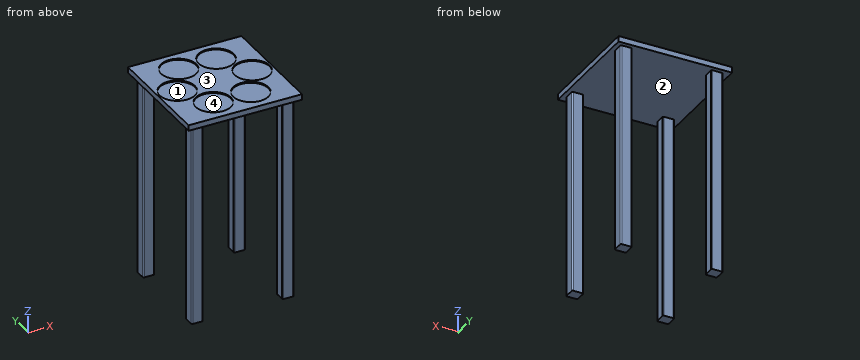
from build123d import *

# Parameters (mm, degrees)
F0_W     = 500
F0_H     = 500
F0_R     = 77.5
F1_DEPTH = 25
F2_DEPTH = 5
F4_DEPTH = 900


with BuildPart() as f1:
    # F0 (on Top) → F1 (new body)
    with BuildSketch(Plane.XY):
        with Locations((0, -2.197117)):
            Rectangle(F0_W, F0_H)
        with Locations((-82.5, -142.894192)):
            Circle(F0_R, mode=Mode.SUBTRACT)
        with Locations((82.5, -142.894192)):
            Circle(F0_R, mode=Mode.SUBTRACT)
        with Locations((-165, 0)):
            Circle(F0_R, mode=Mode.SUBTRACT)
        with Locations((-82.5, 142.894192)):
            Circle(F0_R, mode=Mode.SUBTRACT)
        with Locations((165, 0)):
            Circle(F0_R, mode=Mode.SUBTRACT)
        with Locations((82.5, 142.894192)):
            Circle(F0_R, mode=Mode.SUBTRACT)
        with Locations((-82.5, 142.894192)):
            Circle(F0_R)
        with Locations((82.5, 142.894192)):
            Circle(F0_R)
        with Locations((165, 0)):
            Circle(F0_R)
        with Locations((-165, 0)):
            Circle(F0_R)
        with Locations((-82.5, -142.894192)):
            Circle(F0_R)
        with Locations((82.5, -142.894192)):
            Circle(F0_R)
    extrude(amount=-F1_DEPTH)

    # F0 (on Top) → F2 (cut)
    with BuildSketch(Plane.XY):
        with Locations((-82.5, 142.894192)):
            Circle(F0_R)
        with Locations((82.5, 142.894192)):
            Circle(F0_R)
        with Locations((165, 0)):
            Circle(F0_R)
        with Locations((82.5, -142.894192)):
            Circle(F0_R)
        with Locations((-82.5, -142.894192)):
            Circle(F0_R)
        with Locations((-165, 0)):
            Circle(F0_R)
    extrude(amount=-F2_DEPTH, mode=Mode.SUBTRACT)

    # F3 (on face) → F4 (join)
    with BuildSketch(Plane(origin=(0, 0, -25), x_dir=(1, 0, 0), z_dir=(0, 0, -1))):
        with BuildLine():
            ThreePointArc((225, 172.197117), (228.535534, 173.661583), (230, 177.197117))
            Line((230, 177.197117), (230, 217.197117))
            ThreePointArc((230, 217.197117), (228.535534, 220.732651), (225, 222.197117))
            Line((225, 222.197117), (185, 222.197117))
            ThreePointArc((185, 222.197117), (181.464466, 220.732651), (180, 217.197117))
            Line((180, 217.197117), (180, 177.197117))
            ThreePointArc((180, 177.197117), (181.464466, 173.661583), (185, 172.197117))
            Line((185, 172.197117), (225, 172.197117))
        make_face()
        with BuildLine():
            ThreePointArc((-175, 172.197117), (-171.464466, 173.661583), (-170, 177.197117))
            Line((-170, 177.197117), (-170, 217.197117))
            ThreePointArc((-170, 217.197117), (-171.464466, 220.732651), (-175, 222.197117))
            Line((-175, 222.197117), (-215, 222.197117))
            ThreePointArc((-215, 222.197117), (-218.535534, 220.732651), (-220, 217.197117))
            Line((-220, 217.197117), (-220, 177.197117))
            ThreePointArc((-220, 177.197117), (-218.535534, 173.661583), (-215, 172.197117))
            Line((-215, 172.197117), (-175, 172.197117))
        make_face()
        with BuildLine():
            ThreePointArc((-175, -227.802883), (-171.464466, -226.338417), (-170, -222.802883))
            Line((-170, -222.802883), (-170, -182.802883))
            ThreePointArc((-170, -182.802883), (-171.464466, -179.267349), (-175, -177.802883))
            Line((-175, -177.802883), (-215, -177.802883))
            ThreePointArc((-215, -177.802883), (-218.535534, -179.267349), (-220, -182.802883))
            Line((-220, -182.802883), (-220, -222.802883))
            ThreePointArc((-220, -222.802883), (-218.535534, -226.338417), (-215, -227.802883))
            Line((-215, -227.802883), (-175, -227.802883))
        make_face()
        with BuildLine():
            Line((185, -227.802883), (225, -227.802883))
            ThreePointArc((225, -227.802883), (228.535534, -226.338417), (230, -222.802883))
            Line((230, -222.802883), (230, -182.802883))
            ThreePointArc((230, -182.802883), (228.535534, -179.267349), (225, -177.802883))
            Line((225, -177.802883), (185, -177.802883))
            ThreePointArc((185, -177.802883), (181.464466, -179.267349), (180, -182.802883))
            Line((180, -182.802883), (180, -222.802883))
            ThreePointArc((180, -222.802883), (181.464466, -226.338417), (185, -227.802883))
        make_face()
    extrude(amount=F4_DEPTH)


solid = f1.part
CAD build for the part. Positions are in the model's coordinates, mm. Face numbers are marked on the shaded views. A direction names the side the tool comes from. Round coordinates to 2 decimals unless told otherwise and drop trailing zeros. Order: outer loops, then holes, each group sorted by start corner. A loop starts at its lowest first (then second) coordinate and runs counter-clockwise, first axis right, second up. Notation, with made-up numbers: (-4, 44) -> (17, 44) arc R22 cw to (17, 60) -> close; hole circle Ø2 at (-39.75, 0.5). An arc over 180 degrees is marked (long way). Write each question's results on one line, items separated by ' | '.
1. 3-axis set-ups, long thin cutter, end or side, ignore diameter. For the marked faces 1 and 2: which of +Z, -Z, +X, -X, +Y, -Y reach the whole face in a straight line?
Findings below:
face 1: +Z | face 2: -Z
2. Cut at C-C (x = 149.5). Give the cut face in (y, z).
Findings below:
outline: (-252.2, -25) -> (247.8, -25) -> (247.8, 0) -> (181.85, 0) -> (181.85, -5) -> (103.94, -5) -> (103.94, 0) -> (75.93, 0) -> (75.93, -5) -> (-75.93, -5) -> (-75.93, 0) -> (-103.94, 0) -> (-103.94, -5) -> (-181.85, -5) -> (-181.85, 0) -> (-252.2, 0) -> close
3. Wall check: line 1 along X through (y, z) = (186, -626); line 2 along Y through (x, z) = (-204, -349); line 3 along Y through (x, z) = (82.5, -1.3). Give the ranges that are in metal, low to high. Write a range as [from, to].
Findings below:
line 1: x = [-220, -170], [180, 230] | line 2: y = [-222.2, -172.2], [177.8, 227.8] | line 3: y = [-252.2, -220.39], [-65.39, 65.39], [220.39, 247.8]
4. Cut at D-D (x = -107). Give the cut face in (y, z).
Findings below:
outline: (-252.2, -25) -> (247.8, -25) -> (247.8, 0) -> (216.42, 0) -> (216.42, -5) -> (69.37, -5) -> (69.37, 0) -> (51.4, 0) -> (51.4, -5) -> (-51.4, -5) -> (-51.4, 0) -> (-69.37, 0) -> (-69.37, -5) -> (-216.42, -5) -> (-216.42, 0) -> (-252.2, 0) -> close
5. Cut at A-A (z = -443). Count the separate pieces of the cut face and the enclosed holes in it, plus the area to 3 significant figures.
Findings below:
separate pieces: 4 | enclosed holes: 0 | area: 9,910 mm²
6. Cut at B-B (y = 0). Give the cut face in (x, z).
Findings below:
outline: (-250, -25) -> (250, -25) -> (250, 0) -> (242.5, 0) -> (242.5, -5) -> (87.5, -5) -> (87.5, 0) -> (-87.5, 0) -> (-87.5, -5) -> (-242.5, -5) -> (-242.5, 0) -> (-250, 0) -> close
7. Flat gauge pins, fed straight in: P1, Ø20, axis at y = -198, z = -634, coming from the -X side; P2, Ø12, axis at x = -154, y = -197, coming from the -Z side; P3, Ø12, axis at x = -199.5, z = -402.5, coming from the +Y side. Where does each tip first touch, or does it go through?
Findings below:
P1: stops at x = -220 | P2: stops at z = -25 | P3: stops at y = 227.8
8. Pull direction X, two halves, no side cores. Call the marked faces 3 and 4: pulls with the +X half, pulls with the -X half, needs draft (parallel to the pull), parting line crosses it, or undercut.
Findings below:
face 3: needs draft | face 4: undercut
